from build123d import *

# Parameters (mm, degrees)
SKETCH1_W           = 456.177532672
SKETCH1_H           = 285.75
BOSS_EXTRUDE1_DEPTH = 6.35
CUT_EXTRUDE1_REACH  = 367.675
SKETCH2_W           = 438.651532672
SKETCH2_H           = 152.4
FILLET1_R           = 38.1
HOLE1_D             = 3.175
HOLE1_DEPTH         = 38.1
HOLE1_CSINK_D       = 10.16
HOLE1_CSINK_ANGLE   = 82
HOLE1_TIP           = 0.953866233


with BuildPart() as part:
    # Sketch1 → Boss-Extrude1 (new body)
    with BuildSketch(Plane.XY):
        with Locations((0, -142.875)):
            Rectangle(SKETCH1_W, SKETCH1_H)
    extrude(amount=BOSS_EXTRUDE1_DEPTH)

    # Sketch2 → Cut-Extrude1 (cut, up to next)
    with BuildSketch(Plane.XY.offset(6.35), mode=Mode.PRIVATE) as cut_extrude1_sk1:
        with Locations((0, -142.875)):
            Rectangle(SKETCH2_W, SKETCH2_H)
    cut_extrude1_tool1 = extrude(cut_extrude1_sk1.sketch, amount=-CUT_EXTRUDE1_REACH, mode=Mode.PRIVATE) & part.part
    add(cut_extrude1_tool1.solids().sort_by_distance((0, -142.875, 6.35))[0], mode=Mode.SUBTRACT)

    # Fillet1
    fillet1_edges = [part.edges().sort_by_distance(p)[0] for p in [
        (219.325766336, -66.675, 3.175),
        (219.325766336, -219.075, 3.175),
        (-219.325766336, -219.075, 3.175),
        (-219.325766336, -66.675, 3.175),
    ]]
    fillet(fillet1_edges, radius=FILLET1_R)

    # Hole1
    with Locations(Plane.XY.offset(6.35)):
        with Locations((-218.563766336, -266.7), (-218.563766336, -41.275), (218.563766336, -266.7), (218.563766336, -41.275)):
            CounterSinkHole(HOLE1_D / 2, HOLE1_CSINK_D / 2, depth=HOLE1_DEPTH, counter_sink_angle=HOLE1_CSINK_ANGLE)
            with Locations((0, 0, -(HOLE1_DEPTH + HOLE1_TIP / 2))):  # 118° drill point
                Cone(0, HOLE1_D / 2, HOLE1_TIP, mode=Mode.SUBTRACT)


solid = part.part
Work out the finished part from the listing and answer in its coordinate system (mm). A direction names the side the tool comes from. Coordinates: 2 decimals unless noted, no trailing zeros. Write each loop counter-clockwise with the first axis right and the second up, starting at its lowest first coordinate (ties: lowest second). Pieces come first, ordered by that corner, then holes.
1. The part is cut by section B-B, the plane x = -132.5. Write down the section's boundary in (y, z) (3 decimals).
Results list:
outline: (-285.75, 0) - (-219.075, 0) - (-219.075, 6.35) - (-285.75, 6.35) - close; (-66.675, 0) - (0, 0) - (0, 6.35) - (-66.675, 6.35) - close
2. For a pull along X with two mould halves and no side action, classify faces 3 (the conical face through (216.888, -266.172, 2.527)), 4 (the flat face through (-3, -46, 0)) as +X half, -X half, draft (parallel to the pull), parting line (faces both ways), or undercut.
Results list:
face 3: undercut
face 4: draft
3. For faces 1 (the cylindrical face through (207.87, -208.21, 3.13)), 2 (the conical face through (-216.808, -41.198, 2.527)), determine the directions among +Z, -Z, +X, -X, +Y, -Y from which every point of the face is accessible in a straight line to the end or side of a thin tool.
Results list:
face 1: +Z, -Z
face 2: +Z
4. Consider line 1 along X through (y, z) = (-266.7, 1.75); line 2 along Y through (x, z) = (134.5, 1) (3 decimals); line 3 along X through (y, z) = (-160.5, 5.25). Determine where each line is inside the solid, lowest interval first.
Results list:
line 1: x = -228.09 to -220.15, -216.98 to 216.98, 220.15 to 228.09
line 2: y = -285.75 to -219.075, -66.675 to 0
line 3: x = -228.09 to -219.33, 219.33 to 228.09
5. The part is cut by section A-A, the plane y = -160. Write down the section's boundary in (x, z), and give its area (3 significant figures).
Results list:
outline: (-228.09, 0) - (-219.33, 0) - (-219.33, 6.35) - (-228.09, 6.35) - close; (219.33, 0) - (228.09, 0) - (228.09, 6.35) - (219.33, 6.35) - close
area: 111 mm2
6. The part is cut by section C-C, the plane z = 1. State how many separate pieces and enclosed holes the cut face has, and give its area (3 significant figures).
Results list:
separate pieces: 1
enclosed holes: 5
area: 64,700 mm2
7. A flat-ended cylindrical pin translates along its axis: pin 1 (5 mm diameter, centred on x = -218.56, y = -41.28, fed in from +Z). Find the tip coordinate at first contact, or state that the pin passes through.
Results list:
pin 1: stops at z = 3.39
